```python
from build123d import *

# Parameters (mm, degrees)
F0_W     = 63.896875
F0_H     = 55.959375
F1_DEPTH = 66.675
F2_W     = 63.896875
F2_H     = 55.959375
F3_DEPTH = 3.175
F4_R     = 2.54
F5_DEPTH = 4.7625


# Not quite as in the source:
# - a pattern or mirror of a feature is missing from the dataset's text; its kind, count and spacing are read off the source's solid


with BuildPart() as f1:
    # F0 (on Top) → F1 (new body)
    with BuildSketch(Plane.XY):
        Polygon((35.1234375, -31.1546875), (35.1234375, 31.1546875), (-35.1234375, 31.1546875), (-35.1234375, -31.1546875), align=None)
        Rectangle(F0_W, F0_H, mode=Mode.SUBTRACT)
    extrude(amount=F1_DEPTH)

    # F2 (on Top) → F3 (join)
    with BuildSketch(Plane.XY):
        Rectangle(F2_W, F2_H)
        with BuildLine():
            ThreePointArc((-27.1859375, 6.1708083338), (0, 26.3921875), (27.1859375, 6.1708083338))
            Line((27.1859375, 6.1708083338), (0, -9.525))
            Line((0, -9.525), (-27.1859375, 6.1708083338))
        make_face(mode=Mode.SUBTRACT)
    extrude(amount=F3_DEPTH)

    # F4 (on face) → F5 (join)
    with BuildSketch(Plane.XZ.offset(31.1546875)):
        with BuildLine():
            Line((-35.1234375, 26.9875), (-35.1234375, 39.6875))
            Line((-35.1234375, 39.6875), (-41.4734375, 39.6875))
            ThreePointArc((-41.4734375, 39.6875), (-47.8234375, 33.3375), (-41.4734375, 26.9875))
            Line((-41.4734375, 26.9875), (-35.1234375, 26.9875))
        make_face()
        with Locations((-41.4734375, 33.3375)):
            Circle(F4_R, mode=Mode.SUBTRACT)
    f5 = extrude(amount=-F5_DEPTH)

    # F5_copies: F5 across plane
    add(f5.mirror(Plane(origin=(0, 0, 0), x_dir=(0, 0, 1), z_dir=(1, 0, 0))))


solid = f1.part
```
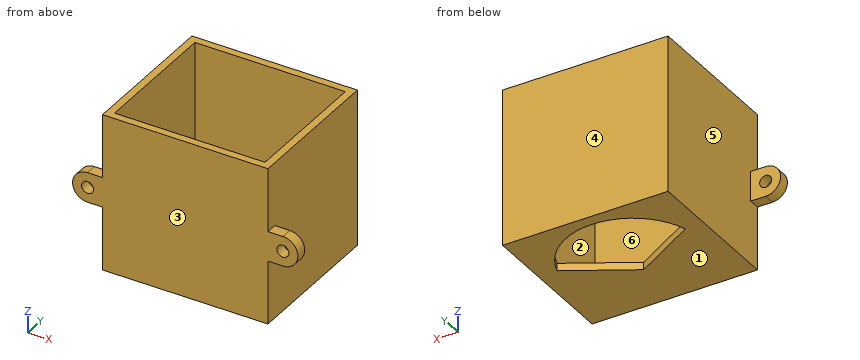
The listing builds one solid part. Answer for the finished solid, in the listing's coordinates (mm). Face numbers are marked on the shaded views. A direction names the side the tool comes from. Coordinates: 2 decimals unless noted, no trailing zeros. Write each loop counter-clockwise with the first axis right and the second up, starting at its lowest first coordinate (ties: lowest second). Pieces come first, ordered by that corner, then holes. Notation, with made-up numbers: M 62.25,51.5 L 99.25,51.5 A31 ccw 99.25,77.5 Z; hole C -24.5,-40 d7. An arc over 180 degrees is marked long. Use a Markdown table: item, result. Add a question column.
1. For a pull along Y with two mould halves and no side action, classify the marked faces 3, 4, 5 and 6 as +Y half, -Y half, draft (parallel to the pull), parting line (faces both ways), or undercut.
2. Given P1, Ø12, axis at y = -9.5, z = 8, coming from the +X side; P2, Ø6.5, axis at x = -41, z = 30.5, coming from the +Y side; P3, Ø1.4, axis at x = -39, y = -29, coming from the -Z side, each flat-ended and moving along its own axis, determine where each tip first touches the part or whether it passes through.
3. Section A-A (z = 54) is taken. Give the vertices of the cut face in (x, y).
4. Which of the six approach directions +Z, -Z, +X, -X, +Y, -Y give full straight-line access (tool end or side, diameter ignored) to the marked faces 1 and 2?
5. Section B-B (y = 18) is taken. Give the vertices of the cut face in (x, z) (3 decimals), plus the area to 3 significant figures.
6. Section C-C (x = 23.5) is taken. Give the vertices of the cut face in (y, z) (3 decimals).
7. Straight lines are drawn through the part: line 1 along Y through (x, z) = (2.5, 27); line 2 along X through (y, z) = (-26, 9); line 3 along Z through (x, y) = (-27.5, 7.5) (3 decimals). For each, find the intervals that lie inside material, in ascending order. Write a range as [from, to].
8. Section D-D (y = -18.5) is taken. Give the vertices of the cut face in (x, z) (3 decimals).
Data:
| question | item | result |
|---|---|---|
| 1 | face 3 | -Y half |
| 1 | face 4 | +Y half |
| 1 | face 5 | draft |
| 1 | face 6 | undercut |
| 2 | P1 | stops at x = 35.12 |
| 2 | P2 | stops at y = -26.39 |
| 2 | P3 | stops at z = 26.99 |
| 3 | outline | M -35.12,-31.15 L 35.12,-31.15 L 35.12,31.15 L -35.12,31.15 Z; hole M -31.95,-27.98 L 31.95,-27.98 L 31.95,27.98 L -31.95,27.98 Z |
| 4 | face 1 | -Z, +X, -X, +Y, -Y |
| 4 | face 2 | +Z |
| 5 | outline | M -35.123,0 L -20.149,0 L -20.149,3.175 L -31.948,3.175 L -31.948,66.675 L -35.123,66.675 Z; M 20.149,0 L 35.123,0 L 35.123,66.675 L 31.948,66.675 L 31.948,3.175 L 20.149,3.175 Z |
| 5 | area | 498 mm2 |
| 6 | outline | M -31.155,0 L 4.043,0 L 4.043,3.175 L -27.98,3.175 L -27.98,66.675 L -31.155,66.675 Z; M 13.928,0 L 31.155,0 L 31.155,66.675 L 27.98,66.675 L 27.98,3.175 L 13.928,3.175 Z |
| 7 | line 1 | y = [-31.15, -27.98], [27.98, 31.15] |
| 7 | line 2 | x = [-35.12, -31.95], [31.95, 35.12] |
| 7 | line 3 | z = [0, 3.175] |
| 8 | outline | M -35.123,0 L 35.123,0 L 35.123,66.675 L 31.948,66.675 L 31.948,3.175 L -31.948,3.175 L -31.948,66.675 L -35.123,66.675 Z |
